Could you check a few things on this model? Use its own coordinates, in mm. A direction names the side the tool comes from. Coordinates: 2 decimals unless noted, no trailing zeros. Write each loop counter-clockwise with the first axis right and the second up, starting at its lowest first coordinate (ties: lowest second). Pieces come first, ordered by that corner, then holes. Notation, with made-up numbers: (-33, 68) - (-15, 68) arc R22 ccw to (-15, 96) - close; hole circle Ø10 at (-27.75, 27). An arc over 180 degrees is marked (long way). Write item = value, one per line. Start each with the question number.
```python
from build123d import *

# Parameters (mm, degrees)
F0_W     = 116.2
F0_H     = 57
F1_DEPTH = 15
F2_T     = -1
F3_DEPTH = 1.001


with BuildPart() as f1:
    # F0 (on Top) → F1 (new body)
    with BuildSketch(Plane.XY):
        with Locations((58.1, -28.5)):
            Rectangle(F0_W, F0_H)
    extrude(amount=F1_DEPTH)

    # F2
    f2_openings = [f1.faces().sort_by_distance(p)[0] for p in [
        (58.1, -28.5, 15),
    ]]
    offset(amount=F2_T, openings=f2_openings)

    # F3 (cut, through all): a face of the model
    f3_faces = [f1.faces().sort_by_distance(p)[0] for p in [
        (58.1, -28.5, 1),
    ]]
    extrude(f3_faces, amount=-F3_DEPTH, mode=Mode.SUBTRACT)


solid = f1.part
```
1) Suppose I cut it at B-B on y = -28. Please give me the cut outline in (x, z), plus the area to 3 significant figures.
2) If I drill on probe 1 along X at (y, z) = (-41.5, 14.25); probe 2 along Y at (x, z) = (71.5, 4.75), over which ranges is the centre line in solid material (lowest first)? Write a range as [from, to].
3) Suppose I cut it at C-C on z = 10.75. Please give me the cut outline in (x, y).
4) Thinking about a two-plate mould opening in Y: for faces 1 (the flat face through (115.2, -29, 8)), 2 (the flat face through (57, -57, 7)), 3 (the flat face through (116.2, -29, 7)), which applies, +Y half, -Y half, draft (parallel to the pull), parting line (faces both ways), or undercut?
5) Suppose I cut it at A-A on x = 70. Please give me the cut outline in (y, z), plus the area to 3 significant figures.
6) Which directions (+Z, -Z, +X, -X, +Y, -Y) give clear straight access to the entire face, cutting with the end or side of a thin tool? Please do faces 4 (the flat face through (0, -29, 7)), 5 (the flat face through (57, -56, 8)).
Reply:
q1.outline = (0, 0) - (1, 0) - (1, 15) - (0, 15) - close; (115.2, 0) - (116.2, 0) - (116.2, 15) - (115.2, 15) - close
q1.area = 30.0 mm^2
q2.probe_1 = [0, 1], [115.2, 116.2]
q2.probe_2 = [-57, -56], [-1, 0]
q3.outline = (0, -57) - (116.2, -57) - (116.2, 0) - (0, 0) - close; hole (1, -56) - (115.2, -56) - (115.2, -1) - (1, -1) - close
q4.face_1 = undercut
q4.face_2 = -Y half
q4.face_3 = draft
q5.outline = (-57, 0) - (-56, 0) - (-56, 15) - (-57, 15) - close; (-1, 0) - (0, 0) - (0, 15) - (-1, 15) - close
q5.area = 30.0 mm^2
q6.face_4 = +Z, -Z, -X, +Y, -Y
q6.face_5 = +Z, -Z
